Read the model definition and answer for the solid it produces. Units are mm, in the model's axes. Face numbers are marked on the shaded views. A direction names the side the tool comes from. Coordinates: 2 decimals unless noted, no trailing zeros. Order: outer loops, then holes, each group sorted by start corner. A loop starts at its lowest first (then second) coordinate and runs counter-clockwise, first axis right, second up. Notation, with made-up numbers: M -25,78 L 34,78 A27 cw 34,103 Z; hole C 18,7.25 d1. An arc over 180 degrees is marked long. Use a Markdown table: item, result. Add a question column.
1) For the marked faces 1, 2 and 3, determine the directions among +Z, -Z, +X, -X, +Y, -Y from which every point of the face is accessible in a straight line to the end or side of a thin tool.
2) Find section D-D on x = -13. Write down the section's boundary in (y, z), plus the area to 3 significant figures.
3) Find section C-C on y = 15. Write down the section's boundary in (x, z).
4) Find section B-B on y = 4. Write down the section's boundary in (x, z).
5) Find section A-A on x = 30. Write down the section's boundary in (y, z).
6) Find the intervals of material crossed by probe 1 along X at (y, z) = (2.5, -5); probe 2 along Z at (x, y) = (-25.4, 43); probe 3 along Z at (x, y) = (30, 4), in increasing order. Write a range as [from, to].
7) Each of these flat-tipped pins is pushed along its axis until it touches: pin 1 Ø7 at (x, z) = (-30, -5) entering from +Y; pin 2 Ø12 at (y, z) = (49.5, -11.5) entering from -X; pin 3 Ø8 at (x, z) = (-17, -11.5) entering from +Y; pin 4 Ø3 at (x, y) = (36.5, 40) entering from -Z. Where does it stop, or does it pass through?
from build123d import *

# Parameters (mm, degrees)
SKETCH1_W                    = 80
SKETCH1_H                    = 30
BOSS_EXTRUDE1_DEPTH          = 55
CSK_FOR_M4_SFHCS1_AT_2_COUNT = 2
CSK_FOR_M4_SFHCS1_AT_2_PITCH = 60
M4X0_7_TAPPED_HOLE1_D        = 3.3
M4X0_7_TAPPED_HOLE1_DEPTH    = 20
M4X0_7_TAPPED_HOLE1_TIP      = 0.991420021
CHAMFER1_SIZE                = 5
SKETCH9_W                    = 80
SKETCH9_H                    = 45
CUT_EXTRUDE1_DEPTH           = 10


with BuildPart() as part:
    # Sketch1 → Boss-Extrude1 (new body)
    with BuildSketch(Plane(origin=(0, 0, 0), x_dir=(1, 0, 0), z_dir=(0, 1, 0))):
        Rectangle(SKETCH1_W, SKETCH1_H)
    extrude(amount=BOSS_EXTRUDE1_DEPTH)

    # Sketch5 → CSK for M4 SFHCS1 (revolve, cut)
    with BuildSketch(Plane(origin=(-30, 55, -5), x_dir=(0, 0, 1), z_dir=(1, 0, 0))):
        Polygon((0, 0), (0, 55), (2.25, 55), (2.25, 47.23), (4.48, 45), (4.48, 0), align=None)
    csk_for_m4_sfhcs1 = revolve(axis=Axis((-30, 61.35, -5), (0, -1, 0)), mode=Mode.SUBTRACT)

    # CSK for M4 SFHCS1 at 2: CSK for M4 SFHCS1 ×2
    with Locations(*[(i * CSK_FOR_M4_SFHCS1_AT_2_PITCH, 0, 0) for i in range(1, CSK_FOR_M4_SFHCS1_AT_2_COUNT)]):
        add(csk_for_m4_sfhcs1, mode=Mode.SUBTRACT)

    # M4x0.7 Tapped Hole1
    with Locations(Plane(origin=(0, 55, 0), x_dir=(1, 0, 0), z_dir=(0, 1, 0))):
        with Locations((-25.4, -4.078), (25.4, -4.078)):
            Hole(M4X0_7_TAPPED_HOLE1_D / 2, depth=M4X0_7_TAPPED_HOLE1_DEPTH)
            with Locations((0, 0, -(M4X0_7_TAPPED_HOLE1_DEPTH + M4X0_7_TAPPED_HOLE1_TIP / 2))):  # 118° drill point
                Cone(0, M4X0_7_TAPPED_HOLE1_D / 2, M4X0_7_TAPPED_HOLE1_TIP, mode=Mode.SUBTRACT)

    # Chamfer1
    chamfer1_edges = [part.edges().sort_by_distance(p)[0] for p in [
        (40, 27.5, 15),
        (-40, 27.5, 15),
    ]]
    chamfer(chamfer1_edges, length=CHAMFER1_SIZE)

    # Sketch9 → Cut-Extrude1 (cut)
    with BuildSketch(Plane(origin=(0, 0, -15), x_dir=(-1, 0, 0), z_dir=(0, 0, -1))):
        with Locations((0, 32.5)):
            Rectangle(SKETCH9_W, SKETCH9_H)
    extrude(amount=-CUT_EXTRUDE1_DEPTH, mode=Mode.SUBTRACT)


solid = part.part
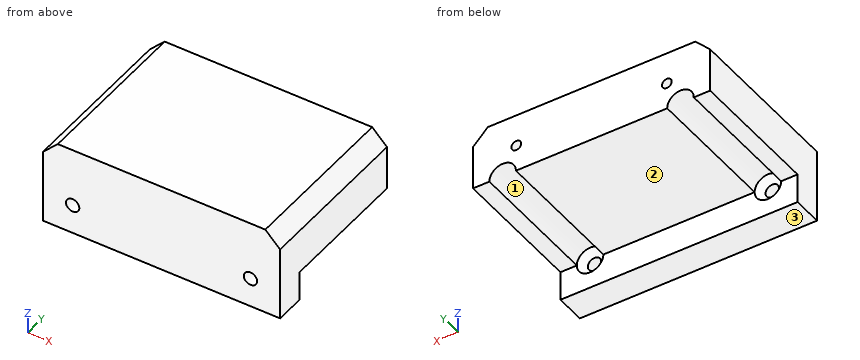
Check result:
| question | item | result |
|---|---|---|
| 1 | face 1 | -Z, +Y |
| 1 | face 2 | -Z, +X, -X, +Y |
| 1 | face 3 | -Z, +X, -X, +Y, -Y |
| 2 | outline | M 0,-15 L 10,-15 L 10,-5 L 55,-5 L 55,15 L 0,15 Z |
| 2 | area | 1,200 mm2 |
| 3 | outline | M -40,-5 L -34.48,-5 A4.48 cw -25.52,-5 L 25.52,-5 A4.48 cw 34.48,-5 L 40,-5 L 40,10 L 35,15 L -35,15 L -40,10 Z |
| 4 | outline | M -40,-15 L 40,-15 L 40,10 L 35,15 L -35,15 L -40,10 Z; hole C -30,-5 d4.5; hole C 30,-5 d4.5 |
| 5 | outline | M 0,-15 L 10,-15 L 10,-9.48 L 7.77,-7.25 L 0,-7.25 Z; M 0,-2.75 L 7.77,-2.75 L 10,-0.52 L 55,-0.52 L 55,15 L 0,15 Z |
| 6 | probe 1 | x = [-40, -32.25], [-27.75, 27.75], [32.25, 40] |
| 6 | probe 2 | z = [-5, 2.43], [5.73, 15] |
| 6 | probe 3 | z = [-15, -7.25], [-2.75, 15] |
| 7 | pin 1 | stops at y = 9.02 |
| 7 | pin 2 | passes through |
| 7 | pin 3 | stops at y = 10 |
| 7 | pin 4 | stops at z = -5 |
